from build123d import *

# Parameters (mm, degrees)
SKETCH1_W                    = 300
SKETCH1_H                    = 300
BOSS_EXTRUDE1_DEPTH          = 3.175
SKETCH2_W                    = 52
SKETCH2_H                    = 40
CUT_EXTRUDE1_DEPTH           = 10
M4_START                     = -3.175
M4_CLEARANCE_HOLE1_OUTLINE_R = 2.15
M4_CLEARANCE_HOLE1_DEPTH     = 3.175
M3_CLEARANCE_HOLE2_D         = 3.2
M2_5_CLEARANCE_HOLE1_D       = 2.7
M3_CLEARANCE_HOLE3_D         = 3.2
M3_CLEARANCE_HOLE4_D         = 3.2
SKETCH14_R                   = 10
CUT_EXTRUDE2_DEPTH           = 10
SKETCH5_W                    = 196
SKETCH5_H                    = 3.2
CUT_EXTRUDE3_DEPTH           = 10


# Read off the part's stored shape, not the designer's step: M4 Clearance Hole1
with BuildPart() as part:
    # Sketch1 → Boss-Extrude1 (new body)
    with BuildSketch(Plane(origin=(0, 0, 0), x_dir=(1, 0, 0), z_dir=(0, 0, -1))):
        with Locations((150, 150)):
            Rectangle(SKETCH1_W, SKETCH1_H)
    extrude(amount=BOSS_EXTRUDE1_DEPTH)

    # Sketch2 → Cut-Extrude1 (cut)
    with BuildSketch(Plane(origin=(0, 0, -3.175), x_dir=(1, 0, 0), z_dir=(0, 0, -1))):
        with Locations((26, 20)):
            Rectangle(SKETCH2_W, SKETCH2_H)
        with Locations((274, 20)):
            Rectangle(SKETCH2_W, SKETCH2_H)
    extrude(amount=-CUT_EXTRUDE1_DEPTH, mode=Mode.SUBTRACT)

    # M4 Clearance Hole1 outline → M4 Clearance Hole1 (cut)
    with BuildSketch(Plane.XY.offset(M4_START)):
        with Locations((266, -226)):
            Circle(M4_CLEARANCE_HOLE1_OUTLINE_R)
        with Locations((216, -76)):
            Circle(M4_CLEARANCE_HOLE1_OUTLINE_R)
        with Locations((216, -226)):
            Circle(M4_CLEARANCE_HOLE1_OUTLINE_R)
        with Locations((266, -76)):
            Circle(M4_CLEARANCE_HOLE1_OUTLINE_R)
    extrude(amount=M4_CLEARANCE_HOLE1_DEPTH, mode=Mode.SUBTRACT)

    # M3 Clearance Hole2 (through all)
    with Locations(Plane(origin=(0, 0, -3.175), x_dir=(-1, 0, 0), z_dir=(0, 0, -1))):
        with Locations((-102, -60), (-10, -157), (-102, -157), (-10, -60)):
            Hole(M3_CLEARANCE_HOLE2_D / 2)

    # M2.5 Clearance Hole1 (through all)
    with Locations(Plane(origin=(0, 0, -3.175), x_dir=(-1, 0, 0), z_dir=(0, 0, -1))):
        with Locations((-102, -186), (-52.6, -250), (-102, -250), (-52.6, -186)):
            Hole(M2_5_CLEARANCE_HOLE1_D / 2)

    # M3 Clearance Hole3 (through all)
    with Locations(Plane(origin=(0, 0, -3.175), x_dir=(-1, 0, 0), z_dir=(0, 0, -1))):
        with Locations((-30, -290), (-270, -290), (-240, -290), (-210, -290), (-180, -290), (-150, -290), (-120, -290), (-90, -290), (-60, -290)):
            Hole(M3_CLEARANCE_HOLE3_D / 2)

    # M3 Clearance Hole4 (through all)
    with Locations(Plane(origin=(0, 0, -3.175), x_dir=(-1, 0, 0), z_dir=(0, 0, -1))):
        with Locations((-72, -10), (-228, -10), (-150, -10)):
            Hole(M3_CLEARANCE_HOLE4_D / 2)

    # Sketch14 → Cut-Extrude2 (cut)
    with BuildSketch(Plane(origin=(0, 0, -3.175), x_dir=(-1, 0, 0), z_dir=(0, 0, -1))):
        with Locations((-82, -171.5)):
            Circle(SKETCH14_R)
    extrude(amount=-CUT_EXTRUDE2_DEPTH, mode=Mode.SUBTRACT)

    # Sketch5 → Cut-Extrude3 (cut)
    with BuildSketch(Plane(origin=(0, 0, -3.175), x_dir=(-1, 0, 0), z_dir=(0, 0, -1))):
        with Locations((-150, -1.6)):
            Rectangle(SKETCH5_W, SKETCH5_H)
    extrude(amount=-CUT_EXTRUDE3_DEPTH, mode=Mode.SUBTRACT)


solid = part.part
Could you check a few things on this model? Use its own coordinates, in mm. Give positions to 0.01 mm unless a question says otherwise; leave off trailing zeros. Order: outer loops, then holes, each group sorted by start corner. A loop starts at its lowest first (then second) coordinate and runs counter-clockwise, first axis right, second up.
1. We'd pull the mould along Y, two halves only. Please class faces 1 (the flat face through (148, -154, 0)), 2 (the cylindrical face through (89.94, -177.58, -1.61)): pulls with the +Y half, pulls with the -Y half, needs draft (parallel to the pull), parting line crosses it, or undercut.
2. Will these pins go through, and if not, where does the flat tip stop? P1, Ø3.5, axis at x = 216, y = -76, coming from the -Z side; P2, Ø1, axis at x = 263, z = -0.5, coming from the +Y side; P3, Ø1.6, axis at y = -23, z = -2, coming from the +X side.
3. Suppose I cut it at A-A (z = -1.3). Give the number of separate pieces and of enclosed holes in the cut face, plus the area to 3 significant figures.
4. I need wall thicknesses on L1, parallel to Y at x = 266, z = -2.15; L2, parallel to X at y = -226, z = -2.6; L3, parallel to Y at x = 102, z = -1.35. Which ranges of each line are inside material? Lowest first, please.
5. Suppose I cut it at B-B (x = 82). List the corners of the cut face in (y, z) for me (3 decimals), plus the area to 3 significant figures.
Solved:
1. face 1: needs draft
1. face 2: undercut
2. P1: passes through
2. P2: stops at y = -40
2. P3: stops at x = 248
3. separate pieces: 1
3. enclosed holes: 25
3. area: 84,700 mm2
4. L1: y = -300 to -228.15, -223.85 to -78.15, -73.85 to -40
4. L2: x = 0 to 213.85, 218.15 to 263.85, 268.15 to 300
4. L3: y = -300 to -251.35, -248.65 to -187.35, -184.65 to -158.6, -155.4 to -61.6, -58.4 to -3.2
5. outline: (-300, -3.175) - (-181.5, -3.175) - (-181.5, 0) - (-300, 0) - close; (-161.5, -3.175) - (-3.2, -3.175) - (-3.2, 0) - (-161.5, 0) - close
5. area: 879 mm2
